Part model, mm, in its own coordinate system. Face numbers are marked on the shaded views. Give positions to 0.01 mm unless a question says otherwise; leave off trailing zeros. Write each loop counter-clockwise with the first axis right and the second up, starting at its lowest first coordinate (ties: lowest second). Pieces come first, ordered by that corner, then holes. Notation, with made-up numbers: M -38,24 L 18,24 A28 cw 18,60 Z; hole C -38,36.25 d5. An arc over 180 degrees is marked long. Answer as CSV lines item,"result". Start each with the question number.
Item 1: Band-saw the part on A-A, the plane y = 78. List the corners of the cut face in (x, z), then the cut area to 3 significant figures.
Item 2: Pin check, flat tips, straight feed: pin 1 (1.5 mm diameter, centred on x = 26, z = -163.5, fed in from +Y); pin 2 (1.5 mm diameter, centred on x = -49.5, z = 133, fed in from +Y); pin 3 (1 mm diameter, centred on x = -170.5, y = 95.5, fed in from -Z). Stop position of each tip, or through.
Item 3: Two-plate mould, pull along Z, no slides. Class the marked faces 1, 2, 3 and 4: +Z half, -Z half, draft (parallel to the pull), parting line (faces both ways), or undercut.
Item 4: Wall check: L1, parallel to Y at x = -33, z = 81.5; L2, parallel to X at y = 502.7, z = 0; L3, parallel to X at y = 406, z = 69.5. Give the ranges that are in metal, low to high. Write a range as from..to.
from build123d import *

# Parameters (mm, degrees)
BOSS_EXTRUDE2_DEPTH = 304.8
CUT_EXTRUDE1_DEPTH  = 304.8
BOSS_EXTRUDE3_DEPTH = 3.048
SKETCH11_R          = 76.2
CUT_EXTRUDE2_DEPTH  = 3.048
BOSS_EXTRUDE4_DEPTH = 3.048


with BuildPart() as part:
    # Sketch4 → Boss-Extrude2 (new body)
    with BuildSketch(Plane(origin=(0, 0, 0), x_dir=(1, 0, 0), z_dir=(0, 1, 0))):
        Polygon((263.964543073, 0), (131.982271537, 228.6), (-131.982271537, 228.6), (-263.964543073, 0), (-131.982271537, -228.6), (131.982271537, -228.6), align=None)
    extrude(amount=BOSS_EXTRUDE2_DEPTH)

    # Sketch5 → section 0 of loft1
    with BuildSketch(Plane(origin=(0, 503.936, 0), x_dir=(1, 0, 0), z_dir=(0, 1, 0)), mode=Mode.PRIVATE) as loft1_s0:
        with BuildLine():
            Line((134.493, 0), (67.2465, 116.474354631))
            Line((67.2465, 116.474354631), (-67.2465, 116.474354631))
            Line((-67.2465, 116.474354631), (-134.493, 0))
            Line((-134.493, 0), (-67.2465, -116.474354631))
            Line((-67.2465, -116.474354631), (67.2465, -116.474354631))
            Line((67.2465, -116.474354631), (134.493, 0))
        make_face()
    # loft up to a face of the part (loft1)
    loft([loft1_s0.sketch, part.faces().sort_by_distance((0, 304.8, 0))[0]])

    # Sketch7 → Cut-Extrude1 (cut)
    with BuildSketch(Plane(origin=(0, 0, 0), x_dir=(-1, 0, 0), z_dir=(0, -1, 0))):
        Polygon((-260.445015833, 0), (-130.222507916, -225.552), (130.222507916, -225.552), (260.445015833, 0), (130.222507916, 225.552), (-130.222507916, 225.552), align=None)
    extrude(amount=-CUT_EXTRUDE1_DEPTH, mode=Mode.SUBTRACT)

    # Sketch8 → section 0 of cut_loft2
    with BuildSketch(Plane(origin=(0, 503.936, 0), x_dir=(1, 0, 0), z_dir=(0, 1, 0)), mode=Mode.PRIVATE) as cut_loft2_s0:
        with BuildLine():
            Line((130.973472817, 0), (65.486736408, 113.426354681))
            Line((65.486736408, 113.426354681), (-65.486736408, 113.426354681))
            Line((-65.486736408, 113.426354681), (-130.973472817, 0))
            Line((-130.973472817, 0), (-65.486736408, -113.426354681))
            Line((-65.486736408, -113.426354681), (65.486736408, -113.426354681))
            Line((65.486736408, -113.426354681), (130.973472817, 0))
        make_face()
    # loft up to a face of the part (cut_loft2)
    loft([cut_loft2_s0.sketch, part.faces().sort_by_distance((0, 304.8, 0))[0]], mode=Mode.SUBTRACT)

    # Sketch10 → Boss-Extrude3 (add)
    with BuildSketch(Plane(origin=(0, 503.936, 0), x_dir=(1, 0, 0), z_dir=(0, 1, 0))):
        Polygon((134.493, 0), (67.2465, 116.474354631), (-67.2465, 116.474354631), (-134.493, 0), (-67.2465, -116.474354631), (67.2465, -116.474354631), align=None)
    extrude(amount=-BOSS_EXTRUDE3_DEPTH)

    # Sketch11 → Cut-Extrude2 (cut)
    with BuildSketch(Plane(origin=(0, 503.936, 0), x_dir=(1, 0, 0), z_dir=(0, 1, 0))):
        with Locations(Location((0, 0, 0), (0, 0, 270))):
            Circle(SKETCH11_R)
    extrude(amount=-CUT_EXTRUDE2_DEPTH, mode=Mode.SUBTRACT)

    # Sketch13 → Boss-Extrude4 (add)
    with BuildSketch(Plane(origin=(0, 0, 0), x_dir=(-1, 0, 0), z_dir=(0, -1, 0))):
        Polygon((-260.445015833, 0), (-130.222507916, -225.552), (130.222507916, -225.552), (260.445015833, 0), (130.222507916, 225.552), (-130.222507916, 225.552), align=None)
    extrude(amount=-BOSS_EXTRUDE4_DEPTH)


solid = part.part
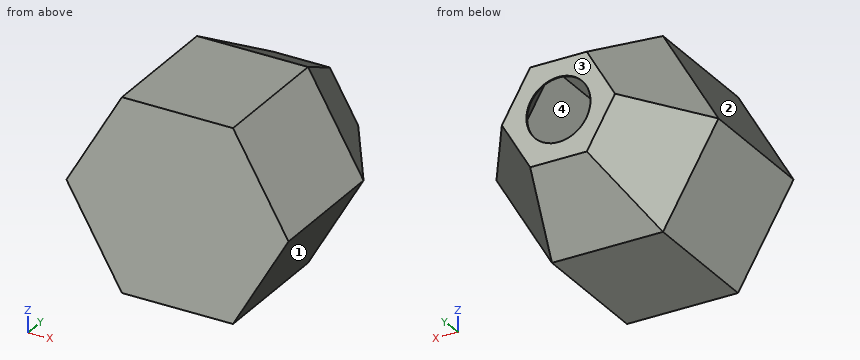
Output:
1,outline,"M -263.96,0 L -131.98,-228.6 L 131.98,-228.6 L 263.96,0 L 131.98,228.6 L -131.98,228.6 Z; hole M -260.45,0 L -130.22,-225.55 L 130.22,-225.55 L 260.45,0 L 130.22,225.55 L -130.22,225.55 Z"
1,area,"4,800 mm²"
2,pin 1,"y = 421.75"
2,pin 2,"y = 475.92"
2,pin 3,"z = -162.75"
3,face 1,"-Z half"
3,face 2,"+Z half"
3,face 3,"draft"
3,face 4,"undercut"
4,L1,"0..3.05, 500.89..503.94"
4,L2,"-135.3..-76.2, 76.2..135.3"
4,L3,"-158.04..-154.52, 154.52..158.04"
